Input: part model. Units: mm. Frame: model coordinates. Give positions to 0.01 mm unless a question says otherwise; leave off trailing zeros. Order: outer loops, then holes, each group sorted by start corner. A loop starts at its lowest first (then second) coordinate and runs counter-clockwise, first axis right, second up. Notation, with made-up numbers: (-29, 84) - (-7, 84) arc R9 cw to (-7, 93) - close; hole circle Ø5 at (76, 75.25). An arc over 180 degrees is marked (long way). Use a Markdown table: item, result.
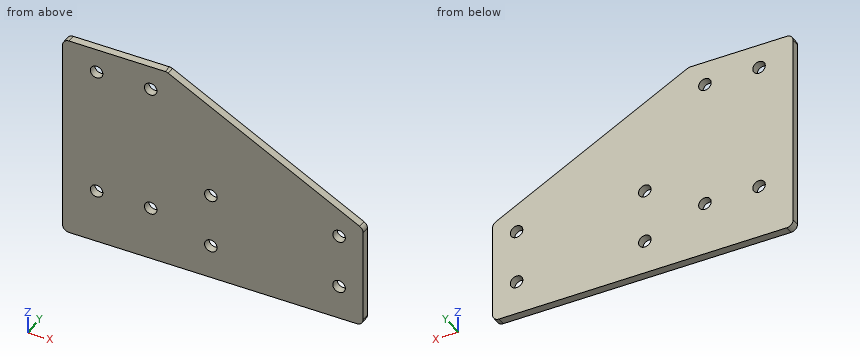
from build123d import *

# Parameters (mm, degrees)
F0_R     = 4.9657
F1_DEPTH = 6.35
F2_R     = 5.08


# Not quite as in the source:
# - a feature names something its author has since deleted; it is built from what else it names


with BuildPart() as f1:
    # F0 (on Front) → F1 (new body)
    with BuildSketch(Plane.XZ):
        Polygon((-96.7471700311, 0.2120000629), (141.3778299689, 0.2120000629), (141.3778299689, 82.7620000629), (-14.1971700311, 163.7245000629), (-96.7471700311, 163.7245000629), (-96.7471700311, 144.6745000629), align=None)
        with Locations((20.7278299689, 27.1995000629)):
            Circle(F0_R, mode=Mode.SUBTRACT)
        with Locations((-69.7596700311, 43.0745000629)):
            Circle(F0_R, mode=Mode.SUBTRACT)
        with Locations((-26.8971700311, 43.0745000629)):
            Circle(F0_R, mode=Mode.SUBTRACT)
        with Locations((20.7278299689, 70.0620000629)):
            Circle(F0_R, mode=Mode.SUBTRACT)
        with Locations((122.3278299689, 27.1995000629)):
            Circle(F0_R, mode=Mode.SUBTRACT)
        with Locations((122.3278299689, 70.0620000629)):
            Circle(F0_R, mode=Mode.SUBTRACT)
        with BuildLine():
            ThreePointArc((-64.7939700311, 144.6745000629), (-69.7596700311, 139.7088000629), (-74.7253700311, 144.6745000629))
            ThreePointArc((-74.7253700311, 144.6745000629), (-69.7596700311, 149.6402000629), (-64.7939700311, 144.6745000629))
        make_face(mode=Mode.SUBTRACT)
        with Locations((-26.8971700311, 144.6745000629)):
            Circle(F0_R, mode=Mode.SUBTRACT)
    extrude(amount=F1_DEPTH)

    # F2
    f2_edges = [f1.edges().sort_by_distance(p)[0] for p in [
        (-96.74717, -3.175, 0.212),
        (-96.74717, -3.175, 163.7245),
        (-14.19717, -3.175, 163.7245),
        (141.37783, -3.175, 82.762),
        (141.37783, -3.175, 0.212),
    ]]
    fillet(f2_edges, radius=F2_R)


solid = f1.part
1. Material intervals for line 1 along Z through (x, y) = (19, -2); line 2 along Z through (x, y) = (17, -0.75); line 3 along X through (y, z) = (-5, 147.5), sorted ascending.
Response:
| item | result |
|---|---|
| line 1 | z = 0.21 to 22.54, 31.85 to 65.41, 74.72 to 146.45 |
| line 2 | z = 0.21 to 23.92, 30.48 to 66.78, 73.34 to 147.49 |
| line 3 | x = -96.75 to -73.84, -65.68 to -30.98, -22.81 to 16.98 |
2. Section query C-C (z = 97.5). Return loops of the section in (x, y), then the cut area to 3 significant figures.
Response:
| item | result |
|---|---|
| outline | (-96.75, -6.35) - (113.06, -6.35) - (113.06, 0) - (-96.75, 0) - close |
| area | 1,330 mm^2 |
3. Pin query (flat end, axial travel): pin 1 (13 mm diameter, centred on x = 122.33, z = 70.06, fed in from +Y); pin 2 (2 mm diameter, centred on x = 36.5, y = -2, fed in from +Z). Return the tip coordinate at first contact, or that it passes through.
Response:
| item | result |
|---|---|
| pin 1 | stops at y = 0 |
| pin 2 | stops at z = 137.86 |
4. Section query B-B (x = 95). Return loops of the section in (y, z), then the cut area to 3 significant figures.
Response:
| item | result |
|---|---|
| outline | (-6.35, 0.21) - (0, 0.21) - (0, 106.9) - (-6.35, 106.9) - close |
| area | 677 mm^2 |
5. Section query A-A (y = -2.75). State how many separate pieces and enclosed holes the cut face has, then the cut area to 3 significant figures.
Response:
| item | result |
|---|---|
| separate pieces | 1 |
| enclosed holes | 8 |
| area | 32,000 mm^2 |
